Input: part model. Units: mm. Frame: model coordinates. Face numbers are marked on the shaded views. Round coordinates to 2 decimals unless told otherwise and drop trailing zeros. Write each loop counter-clockwise with the first axis right and the second up, starting at its lowest first coordinate (ties: lowest second). Pieces come first, ordered by that corner, then holes. Notation, with made-up numbers: (43.5, 17) - (47.5, 17) arc R21 cw to (47.5, 39) - close; hole circle Ø10 at (43.25, -10). An arc over 180 degrees is marked (long way). Use one line per item in the form item = value.
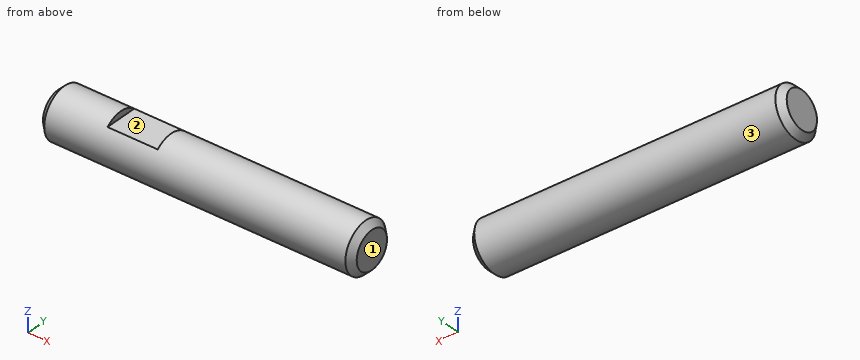
```python
from build123d import *

# Parameters (mm, degrees)
ENL_V_MAT_EXTRU_1_DEPTH      = 4
ENL_V_MAT_EXTRU_1_DEPTH_BACK = 4
ESQUISSE2_W                  = 4
ESQUISSE2_H                  = 0.5


with BuildPart() as part:
    # Esquisse1 → R_volution1 (revolve)
    with BuildSketch(Plane.XY, mode=Mode.PRIVATE) as r_volution1_sk:
        Polygon((0, 0), (0, 1.5), (0.5, 2), (24.5, 2), (25, 1.5), (25, 0), align=None)
    revolve(r_volution1_sk.sketch.rotate(Axis((25, 0, 0), (-1, 0, 0)), 270), axis=Axis((25, 0, 0), (-1, 0, 0)))

    # Esquisse2 → Enl_v. mat.-Extru.1 (cut, two sides: drawn at the far end of the back side and taken through both)
    with BuildSketch(Plane(origin=(0, 0, 0), x_dir=(1, 0, 0), z_dir=(0, 1, 0)).offset(-ENL_V_MAT_EXTRU_1_DEPTH_BACK)):
        with Locations((7, -1.75)):
            Rectangle(ESQUISSE2_W, ESQUISSE2_H)
    extrude(amount=ENL_V_MAT_EXTRU_1_DEPTH + ENL_V_MAT_EXTRU_1_DEPTH_BACK, mode=Mode.SUBTRACT)


solid = part.part
```
(1) Material intervals for L1, parallel to Y at x = 13.5, z = 1.5; L2, parallel to Z at x = 11, y = 1.6, sorted ascending.
Derived:
L1 = -1.32 to 1.32
L2 = -1.2 to 1.2
(2) Draft query along X for the marked faces 1, 2 and 3. Return one class per face: released by +X, released by -X, zero draft, split by the parting line, or undercut.
Derived:
face_1 = released by +X
face_2 = undercut
face_3 = zero draft
(3) First-contact query: pin 1 Ø2 at (x, z) = (4.5, -1) entering from -Y; pin 2 Ø1 at (x, z) = (21.5, 1.5) entering from -Y; pin 3 Ø0.6 at (y, z) = (-0.5, 2) entering from +X. Flat tips, straight axial feed; report the tip coordinate or a pass-through.
Derived:
pin_1 = -2
pin_2 = -1.73
pin_3 = 24.74
(4) Cut plane B-B on x = 16. Output: boundary loops of the cut face in (y, z), then the cut area to 3 significant figures.
Derived:
outline = circle Ø4 at (0, 0)
area = 12.6 mm^2
(5) Cut plane A-A on y = 0. Output: boundary loops of the cut face in (x, z).
Derived:
outline = (0, -1.5) - (0.5, -2) - (24.5, -2) - (25, -1.5) - (25, 1.5) - (24.5, 2) - (9, 2) - (9, 1.5) - (5, 1.5) - (5, 2) - (0.5, 2) - (0, 1.5) - close
